Study the drawing (mm; zero at the part's minimum x, y, z) and answer. A direction names the side the tool comes from. Give positions to 0.01 mm unless a question says otherwise; leave off trailing zeros. Order: outer loops, then holes, each group sorted by start corner. A loop starts at its lowest first (then second) coordinate and runs counter-clockwise, first axis right, second up. Notation, with made-up numbers: (68, 65) - (121, 65) arc R22 ccw to (121, 93) - close; hole circle Ø7 at (-13.75, 57.25). An arc over 180 degrees is marked (long way). Write each question's results on one line, items separated by ' | '. Start each with the question number.
Q1. For a pull along Z with two mould halves and no side action, classify the marked faces 1, 2 and 3 as +Z half, -Z half, draft (parallel to the pull), parting line (faces both ways), or undercut.
Q2. Find section A-A on x = 24. Give the vertices of the cut face in (y, z), and give its area (3 significant figures).
Q3. Flat-ended cylindrical pins translate along their axes: P1, Ø1.9, axis at y = 4, z = 24, coming from the +X side; P2, Ø4, axis at x = 10, z = 28, coming from the -Y side; P3, Ø1.9, axis at x = 34.5, y = 3.5, coming from the -Z side; P4, Ø1.9, axis at x = 3.5, y = 2.5, coming from the +Z side. Find the tip coordinate at first contact, or state that the pin passes through.
Q4. Find section B-B on z = 20. Give the vertices of the cut face in (x, y).
Q5. Find the intervals of material crossed by line 1 along X through (y, z) = (4.5, 11.5); line 2 along Z through (x, y) = (13, 0.5); line 3 along Z through (x, y) = (2, 2), in increasing order. Write a range as from..to.
Q6. A tool of negligible diameter and unlimited length cuts with its end or side. For the marked faces 4, 5, 6, 7 and 8, from which of +Z, -Z, +X, -X, +Y, -Y can it reach the whole face along a straight path? Write none if from no direction.
Q7. Find section C-C on y = 1.75. Give the vertices of the cut face in (x, z), and give its area (3 significant figures).
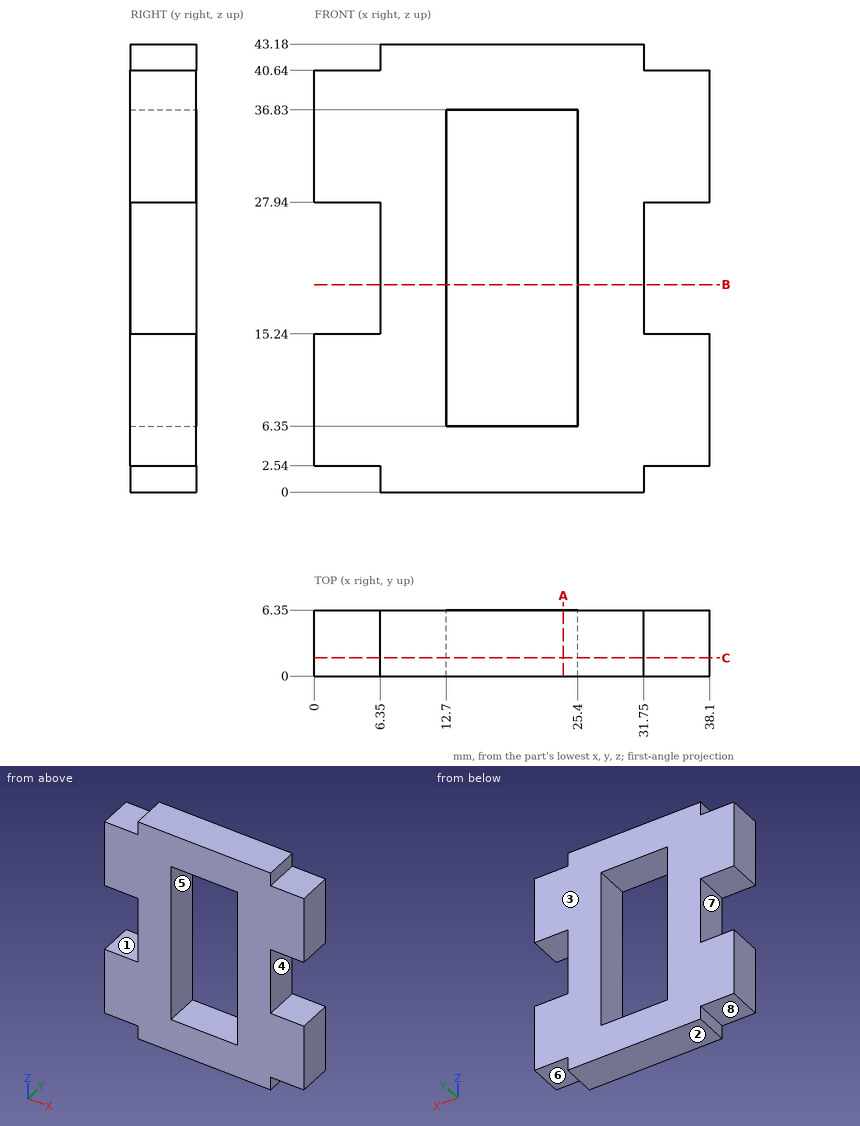
Working result:
1) face 1: undercut | face 2: -Z half | face 3: draft
2) outline: (0, 0) - (6.35, 0) - (6.35, 6.35) - (0, 6.35) - close; (0, 36.83) - (6.35, 36.83) - (6.35, 43.18) - (0, 43.18) - close | area: 80.6 mm²
3) P1: x = 31.75 | P2: y = 0 | P3: z = 2.54 | P4: z = 40.64
4) outline: (6.35, 0) - (12.7, 0) - (12.7, 6.35) - (6.35, 6.35) - close; (25.4, 0) - (31.75, 0) - (31.75, 6.35) - (25.4, 6.35) - close
5) line 1: 0..12.7, 25.4..38.1 | line 2: 0..6.35, 36.83..43.18 | line 3: 2.54..15.24, 27.94..40.64
6) face 4: +X, +Y, -Y | face 5: +Y, -Y | face 6: -Z, +X, +Y, -Y | face 7: -X, +Y, -Y | face 8: -Z, -X, +Y, -Y
7) outline: (0, 2.54) - (6.35, 2.54) - (6.35, 0) - (31.75, 0) - (31.75, 2.54) - (38.1, 2.54) - (38.1, 15.24) - (31.75, 15.24) - (31.75, 27.94) - (38.1, 27.94) - (38.1, 40.64) - (31.75, 40.64) - (31.75, 43.18) - (6.35, 43.18) - (6.35, 40.64) - (0, 40.64) - (0, 27.94) - (6.35, 27.94) - (6.35, 15.24) - (0, 15.24) - close; hole (12.7, 6.35) - (25.4, 6.35) - (25.4, 36.83) - (12.7, 36.83) - close | area: 1,030 mm²
